from build123d import *

# Parameters (mm, degrees)
CROQUIS1_R                  = 52.25
CROQUIS1_R_2                = 12.25
EXTRUIR_L_MINA1_DEPTH       = 64
CROQUIS3_R                  = 80
CROQUIS3_R_2                = 17.25
SALIENTE_EXTRUIR1_DEPTH     = 10
EXTRUIR_L_MINA2_OUTLINE_R   = 51
EXTRUIR_L_MINA2_OUTLINE_R_2 = 31
EXTRUIR_L_MINA2_DEPTH       = 21
EXTRUIR_L_MINA2_2_OUTLINE_R = 31
EXTRUIR_L_MINA2_2_DEPTH     = 5
EXTRUIR_L_MINA2_START       = 16
EXTRUIR_L_MINA2_3_OUTLINE_R = 31
EXTRUIR_L_MINA2_3_DEPTH     = 5
CORTAR_EXTRUIR2_START       = -8
CROQUIS6_R                  = 31
CORTAR_EXTRUIR2_DEPTH       = 8
CORTAR_EXTRUIR4_START       = -23
CROQUIS7_R                  = 12.25
CORTAR_EXTRUIR4_DEPTH       = 23
CROQUIS8_R                  = 7.94
CORTAR_EXTRUIR5_DEPTH       = 10
REDONDEO3_R                 = 3
CORTAR_EXTRUIR6_START       = -40
CROQUIS9_R                  = 17.25
CORTAR_EXTRUIR6_DEPTH       = 40
CROQUIS10_W                 = 24.5
CROQUIS10_H                 = 16
CORTAR_EXTRUIR7_DEPTH       = 42
CROQUIS11_W                 = 24.5
CROQUIS11_H                 = 8
CORTAR_EXTRUIR8_DEPTH       = 42


# Read off the part's stored shape, not the designer's step: Extruir-Lámina2
with BuildPart() as part:
    # Croquis1 → Extruir-Lámina1 (new body)
    with BuildSketch(Plane(origin=(0, 0, 0), x_dir=(1, 0, 0), z_dir=(0, 1, 0))):
        Circle(CROQUIS1_R)
        Circle(CROQUIS1_R_2, mode=Mode.SUBTRACT)
    extrude(amount=EXTRUIR_L_MINA1_DEPTH)

    # Croquis3 → Saliente-Extruir1 (add)
    with BuildSketch(Plane(origin=(0, 0, 0), x_dir=(1, 0, 0), z_dir=(0, 1, 0))):
        with Locations(Location((0, 0, 0), (0, 0, 270))):
            Circle(CROQUIS3_R)
        with Locations(Location((0, 0, 0), (0, 0, 270))):
            Circle(CROQUIS3_R_2, mode=Mode.SUBTRACT)
    extrude(amount=-SALIENTE_EXTRUIR1_DEPTH)

    # Extruir-Lámina2 outline → Extruir-Lámina2 (add)
    with BuildSketch(Plane(origin=(0, 64, 0), x_dir=(1, 0, 0), z_dir=(0, 1, 0))):
        Circle(EXTRUIR_L_MINA2_OUTLINE_R)
        Circle(EXTRUIR_L_MINA2_OUTLINE_R_2, mode=Mode.SUBTRACT)
    extrude(amount=EXTRUIR_L_MINA2_DEPTH)

    # Extruir-L_mina2 2 outline → Extruir-L_mina2 2 (add)
    with BuildSketch(Plane(origin=(0, 64, 0), x_dir=(1, 0, 0), z_dir=(0, 1, 0))):
        Circle(EXTRUIR_L_MINA2_2_OUTLINE_R)
    extrude(amount=EXTRUIR_L_MINA2_2_DEPTH)

    # Extruir-L_mina2 3 outline → Extruir-L_mina2 3 (add)
    with BuildSketch(Plane(origin=(0, 64, 0), x_dir=(1, 0, 0), z_dir=(0, 1, 0)).offset(EXTRUIR_L_MINA2_START)):
        Circle(EXTRUIR_L_MINA2_3_OUTLINE_R)
    extrude(amount=EXTRUIR_L_MINA2_3_DEPTH)

    # Croquis6 → Cortar-Extruir2 (cut)
    with BuildSketch(Plane(origin=(0, 85, 0), x_dir=(1, 0, 0), z_dir=(0, 1, 0)).offset(CORTAR_EXTRUIR2_START)):
        with Locations(Location((0, 0, 0), (0, 0, 270))):
            Circle(CROQUIS6_R)
    extrude(amount=CORTAR_EXTRUIR2_DEPTH, mode=Mode.SUBTRACT)

    # Croquis7 → Cortar-Extruir4 (cut)
    with BuildSketch(Plane(origin=(0, 69, 0), x_dir=(1, 0, 0), z_dir=(0, 1, 0)).offset(CORTAR_EXTRUIR4_START)):
        with Locations(Location((0, 0, 0), (0, 0, 270))):
            Circle(CROQUIS7_R)
    extrude(amount=CORTAR_EXTRUIR4_DEPTH, mode=Mode.SUBTRACT)

    # Croquis8 → Cortar-Extruir5 (cut)
    with BuildSketch(Plane(origin=(0, 0, 0), x_dir=(1, 0, 0), z_dir=(0, 1, 0))):
        with Locations(Location((0, 65, 0), (0, 0, 270))):
            Circle(CROQUIS8_R)
        with Locations(Location((65, 0, 0), (0, 0, 270))):
            Circle(CROQUIS8_R)
        with Locations(Location((0, -65, 0), (0, 0, 270))):
            Circle(CROQUIS8_R)
        with Locations(Location((-65, 0, 0), (0, 0, 270))):
            Circle(CROQUIS8_R)
    extrude(amount=-CORTAR_EXTRUIR5_DEPTH, mode=Mode.SUBTRACT)

    # Redondeo3
    redondeo3_edges = [part.edges().sort_by_distance(p)[0] for p in [
        (-52.25, 0, 0),
    ]]
    fillet(redondeo3_edges, radius=REDONDEO3_R)

    # Croquis9 → Cortar-Extruir6 (cut)
    with BuildSketch(Plane(origin=(0, -10, 0), x_dir=(-1, 0, 0), z_dir=(0, -1, 0)).offset(CORTAR_EXTRUIR6_START)):
        with Locations(Location((0, 0, 0), (0, 0, 270))):
            Circle(CROQUIS9_R)
    extrude(amount=CORTAR_EXTRUIR6_DEPTH, mode=Mode.SUBTRACT)

    # Croquis10 → Cortar-Extruir7 (cut)
    with BuildSketch(Plane(origin=(38.228136726, 0, 35.618423077), x_dir=(0.6816923076923129, 0, -0.7316389803947908), z_dir=(0.7316389803947908, 0, 0.6816923076923129))):
        with Locations((-0.249897299, 21)):
            Rectangle(CROQUIS10_W, CROQUIS10_H)
    extrude(amount=-CORTAR_EXTRUIR7_DEPTH, mode=Mode.SUBTRACT)

    # Croquis11 → Cortar-Extruir8 (cut)
    with BuildSketch(Plane(origin=(38.228136726, 0, 35.618423077), x_dir=(0.6816923076923129, 0, -0.7316389803947908), z_dir=(0.7316389803947908, 0, 0.6816923076923129))):
        with Locations((-0.249897299, 9)):
            Rectangle(CROQUIS11_W, CROQUIS11_H)
    extrude(amount=-CORTAR_EXTRUIR8_DEPTH, mode=Mode.SUBTRACT)


solid = part.part
Could you check a few things on this model? Use its own coordinates, in mm. A direction names the side the tool comes from. Give positions to 0.01 mm unless a question says otherwise; leave off trailing zeros. Order: outer loops, then holes, each group sorted by start corner. A loop starts at its lowest first (then second) coordinate and runs counter-clockwise, first axis right, second up.
Item 1: If we section it at A-A, the plane z = 65: Write out the boundary of the cut face in (x, y).
Item 2: If we mould it in two halves opening along X, with no side actions, what happens to faces 1 (the face through (1, -10, -19)), 2 (the face through (-11.66, 10.28, -12.71)), 3 (the face through (31.514, 16.832, 12.961)), 4 (the face through (-78.1, -4.93, -17.34))? For each: pulls with the +X half, pulls with the -X half, needs draft (parallel to the pull), parting line crosses it, or undercut.
Item 3: I'm going to push flat-ended pins straight in: pin 1 (3 mm diameter, centred on x = 10, y = 66, fed in from +Z); pin 2 (2 mm diameter, centred on x = 11, y = 17.5, fed in from -Z); pin 3 (2 mm diameter, centred on y = 74, z = -1, fed in from +X); pin 4 (12.5 mm diameter, centred on x = 65, z = 0, fed in from -Y). Where does each tip first touch, or does it pass through?
Item 4: If we section it at C-C, the plane y = 44: Write out the boundary of the cut face in (x, z), plus the area to 3 significant figures.
Item 5: If we section it at B-B, the plane x = -65: Write out the boundary of the cut face in (y, z).
Item 6: I need wall thicknesses on line 1 (X direction, y = -4.5, z = 0); line 2 (Z direction, x = 0, y = 79.75); line 3 (X direction, y = 54, z = 0.5). Which ranges of each line are inside material? Lowest first, please.
Item 7: If we section it at D-D, the plane y = 18.5: Write out the boundary of the cut face in (x, z), plus the area to 3 significant figures.
Item 8: For faces 5 (the face through (23, 29, 22)), 6 (the face through (-52.2, 0, -18.9)), 7 (the face through (2.385, -4.93, 72.573)), 8 (the face through (4, 30, -12)), which set-ups out of +Z, -Z, +X, -X, +Y, -Y let a thin tool reach every point of the face, with its end or its side?
Values:
1. outline: (-46.64, -10) - (-7.94, -10) - (-7.94, 0) - (-46.64, 0) - close; (7.94, -10) - (46.64, -10) - (46.64, 0) - (7.94, 0) - close
2. face 1: needs draft
2. face 2: undercut
2. face 3: undercut
2. face 4: parting line crosses it
3. pin 1: stops at z = 50.29
3. pin 2: stops at z = -51.28
3. pin 3: stops at x = 51
3. pin 4: passes through
4. outline: circle Ø104.5 at (0, 0); hole circle Ø24.5 at (0, 0)
4. area: 8,110 mm2
5. outline: (-10, -46.64) - (0, -46.64) - (0, -7.94) - (-10, -7.94) - close; (-10, 7.94) - (0, 7.94) - (0, 46.64) - (-10, 46.64) - close
6. line 1: x = -80 to -72.94, -57.06 to -17.25, 17.25 to 57.06, 72.94 to 80
6. line 2: z = -51 to -31, 31 to 51
6. line 3: x = -52.25 to -12.24, 12.24 to 52.25
7. outline: (0.18, 17.25) - (28.6, 43.73) arc R52.25 ccw (long way) to (45.39, 25.89) - (17.25, -0.33) arc R17.25 cw (long way) to start
7. area: 6,760 mm2
8. face 5: none
8. face 6: +Y
8. face 7: +Y, -Y
8. face 8: -Y
